from build123d import *

# Parameters (mm, degrees)
SKETCH1_R           = 10
SKETCH1_R_2         = 2.5
BOSS_EXTRUDE1_DEPTH = 6.35
BOSS_EXTRUDE2_DEPTH = 6.35
CIRPATTERN1_COUNT   = 25


with BuildPart() as part:
    # Sketch1 → Boss-Extrude1 (new body)
    with BuildSketch(Plane.XY):
        Circle(SKETCH1_R)
        Circle(SKETCH1_R_2, mode=Mode.SUBTRACT)
    extrude(amount=BOSS_EXTRUDE1_DEPTH)

    # Sketch2 → Boss-Extrude2 (add)
    with BuildSketch(Plane.XY.offset(6.35)):
        Polygon((-0.5, 11), (0.5, 11), (1, 9), (-1, 9), align=None)
    boss_extrude2 = extrude(amount=-BOSS_EXTRUDE2_DEPTH)

    # CirPattern1: Boss-Extrude2 ×25 about axis
    cirpattern1_axis = Axis((0, 0, 0), (0, 0, 1))
    for i in range(1, CIRPATTERN1_COUNT):
        add(boss_extrude2.rotate(cirpattern1_axis, i * 360 / CIRPATTERN1_COUNT))


solid = part.part
Read the model definition and answer for the solid it produces. Units are mm, in the model's axes. A direction names the side the tool comes from. Give positions to 0.01 mm unless a question says otherwise; leave off trailing zeros. Write each loop counter-clockwise with the first axis right and the second up, starting at its lowest first coordinate (ties: lowest second). Pieces come first, ordered by that corner, then holes. Notation, with made-up numbers: (80.5, 1.5) - (102.5, 1.5) arc R13 ccw to (102.5, 25.5) - close; hole circle Ø9 at (74, 32). An arc over 180 degrees is marked (long way). Return JSON: item names as keys, results as strings.
Q1. Consider line 1 along Y through (x, z) = (0, 2); line 2 along X through (y, z) = (9.5, 4); line 3 along X through (y, z) = (-6.5, 6). Determine where each line is inside the solid, lowest interval first. Write a range as [from, to].
Reply:
{"line 1": "[-10, -2.5], [2.5, 11]", "line 2": "[-5.55, -4.51], [-3.21, 3.21], [4.51, 5.55]", "line 3": "[-8.7, 8.7]"}
Q2. For a pull along Y with two mould halves and no side action, classify faces 1 (the face through (3.688, 9.295, 3.131)), 2 (the face through (10.19, -2.58, 3.22)), 3 (the face through (5.604, 8.893, 3.219)), 4 (the face through (3.28, -9.99, 3.22)) as released by +Y, released by -Y, zero draft, split by the parting line, or undercut.
Reply:
{"face 1": "released by +Y", "face 2": "undercut", "face 3": "undercut", "face 4": "released by -Y"}
Q3. For faces 5 (the face through (-9.79, 3.84, 3.22)), 6 (the face through (10.173, 2.646, 3.219)), 7 (the face through (-6.675, -8.12, 3.219)), 8 (the face through (1.995, 10.306, 3.219)), 9 (the face through (6.471, -8.895, 3.219)), determine the directions among +Z, -Z, +X, -X, +Y, -Y from which every point of the face is accessible in a straight line to the end or side of a thin tool.
Reply:
{"face 5": "+Z, -Z", "face 6": "+Z, -Z, +X", "face 7": "+Z, -Z, -X", "face 8": "+Z, -Z, +Y", "face 9": "+Z, -Z, +X, -Y"}
Q4. A cutting plane is placed at A-A, the plane x = 0. Determine the outline of the cut face in (y, z).
Reply:
{"outline": "(-10, 0) - (-2.5, 0) - (-2.5, 6.35) - (-10, 6.35) - close; (2.5, 0) - (11, 0) - (11, 6.35) - (2.5, 6.35) - close"}
Q5. Given P1, Ø1.5, axis at y = 6, z = 3.5, coming from the -X side; P2, Ø1, axis at y = -3, z = 3, coming from the -X side, each flat-ended and moving along its own axis, determine where each tip first touches the part or whether it passes through.
Reply:
{"P1": "x = -9.56", "P2": "x = -10.72"}
